Source: CAD feature listing. Evaluate the final solid. Frame: model axes, mm. Face numbers are marked on the shaded views. A direction names the side the tool comes from. Round coordinates to 2 decimals unless told otherwise and drop trailing zeros. Loops run counter-clockwise (first coordinate to the right, second up) from the corner with the lowest first, then second, coordinate; pieces in that order, holes last. Notation, with made-up numbers: (-4, 87.5) - (53, 87.5) arc R26 ccw to (53, 122.5) - close; hole circle Ø3 at (1.5, 52). An arc over 180 degrees is marked (long way). One line per question, with ' | ' between items.
from build123d import *

# Parameters (mm, degrees)
F1_DEPTH = 292.1
F3_DEPTH = 41.276
F4_R     = 5.159375
F5_DEPTH = 4.7625
F6_R     = 5.159375
F7_DEPTH = 4.7625


with BuildPart() as f1:
    # F0 (on Front) → F1 (new body)
    with BuildSketch(Plane.XZ):
        with BuildLine():
            Line((0, 4.7625), (0, 0))
            Line((0, 0), (34.925, 0))
            ThreePointArc((34.925, 0), (39.415128, 1.859872), (41.275, 6.35))
            Line((41.275, 6.35), (41.275, 136.525))
            ThreePointArc((41.275, 136.525), (39.415128, 141.015128), (34.925, 142.875))
            Line((34.925, 142.875), (0, 142.875))
            Line((0, 142.875), (0, 138.1125))
            Line((0, 138.1125), (30.1625, 138.1125))
            ThreePointArc((30.1625, 138.1125), (34.652628, 136.252628), (36.5125, 131.7625))
            Line((36.5125, 131.7625), (36.5125, 11.1125))
            ThreePointArc((36.5125, 11.1125), (34.652628, 6.622372), (30.1625, 4.7625))
            Line((30.1625, 4.7625), (0, 4.7625))
        make_face()
    extrude(amount=F1_DEPTH)

    # F2 (on face) → F3 (cut, through all)
    with BuildSketch(Plane.YZ.offset(41.275)):
        with BuildLine():
            Line((-95.25, 22.225), (-95.25, 0))
            Line((-95.25, 0), (-42.8625, 0))
            Line((-42.8625, 0), (-42.8625, 22.225))
            ThreePointArc((-42.8625, 22.225), (-44.722372, 26.715128), (-49.2125, 28.575))
            Line((-49.2125, 28.575), (-88.9, 28.575))
            ThreePointArc((-88.9, 28.575), (-93.390128, 26.715128), (-95.25, 22.225))
        make_face()
    extrude(amount=-F3_DEPTH, mode=Mode.SUBTRACT)

    # F4 (on face) → F5 (cut, through all)
    with BuildSketch(Plane.XY.offset(142.875)):
        with Locations((19.05, -106.3752)):
            Circle(F4_R)
        with Locations((19.05, -182.5752)):
            Circle(F4_R)
    extrude(amount=-F5_DEPTH, mode=Mode.SUBTRACT)

    # F6 (on face) → F7 (cut, through all)
    with BuildSketch(Plane(origin=(0, 0, 0), x_dir=(1, 0, 0), z_dir=(0, 0, -1))):
        with Locations((19.05, 119.0752)):
            Circle(F6_R)
        with Locations((19.05, 195.2752)):
            Circle(F6_R)
    extrude(amount=-F7_DEPTH, mode=Mode.SUBTRACT)


solid = f1.part
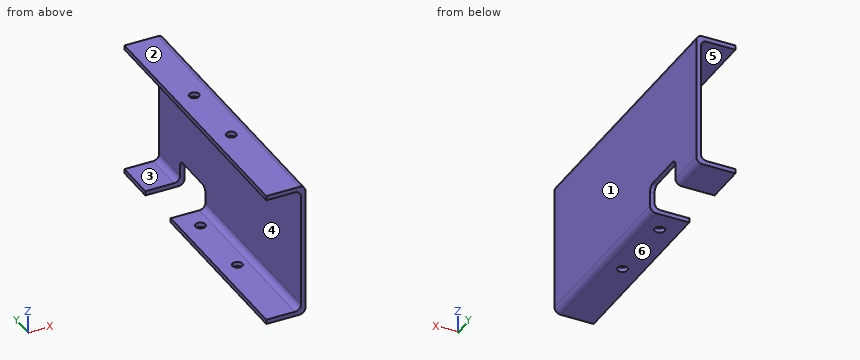
1. Material intervals for probe 1 along Y at (x, z) = (19, 141); probe 2 along Y at (x, z) = (19, 1); probe 3 along Z at (x, y) = (22, -21.5) (1 decimal), sorted ascending.
Worked out:
probe 1: y = -292.1 to -187.73, -177.42 to -111.53, -101.22 to 0 | probe 2: y = -292.1 to -200.43, -190.12 to -124.23, -113.92 to -95.25, -42.86 to 0 | probe 3: z = 0 to 4.8, 138.1 to 142.9
2. Section query C-C, the plane z = 63. Return loops of the section in (x, y) (1 decimal), plus the area to 3 significant figures.
Worked out:
outline: (36.5, -292.1) - (41.3, -292.1) - (41.3, 0) - (36.5, 0) - close | area: 1,390 mm2
3. Contact query for flat-ended pins moving along their axis: P1, Ø6, axis at x = 19.05, y = -195.28, coming from the -Z side; P2, Ø2, axis at y = -122, z = 31, coming from the -X side; P3, Ø18, axis at x = 26, z = 16.5, coming from the -Y side; P4, Ø2.5, axis at x = 38.5, y = -74.5, coming from the -Z side (3 decimals). Output: stop coordinate, or through.
Worked out:
P1: stops at z = 138.11 | P2: stops at x = 36.51 | P3: passes through | P4: stops at z = 28.575
4. Access query for the marked faces 5 and 6. Directions: +Z, -Z, +X, -X, +Y, -Y. A direction counts if a zero-diameter tool reaches every point of the face in a straight line with its end or side. Return the directions, or none.
Worked out:
face 5: -X, +Y, -Y | face 6: -Z, +X, -X, +Y, -Y
5. Section query A-A, the plane x = 19.05. Give the number of separate pieces and of enclosed holes in the cut face, plus the area to 3 significant figures.
Worked out:
separate pieces: 7 | enclosed holes: 0 | area: 2,340 mm2
6. Mould query, pull axis Z, two halves, no side actions, for the marked faces 1, 2, 3 and 4. Classes: released by +Z, released by -Z, zero draft, split by the parting line, or undercut.
Worked out:
face 1: zero draft | face 2: released by +Z | face 3: undercut | face 4: undercut
